Part model, mm, in its own coordinate system. Face numbers are marked on the shaded views. Round coordinates to 2 decimals unless told otherwise and drop trailing zeros. Write each loop counter-clockwise with the first axis right and the second up, starting at its lowest first coordinate (ties: lowest second). Pieces come first, ordered by that corner, then holes.
```python
from build123d import *

# Parameters (mm, degrees)
F0_R     = 13.45
F1_DEPTH = 3


with BuildPart() as f1:
    # F0 (on Front) → F1 (new body)
    with BuildSketch(Plane.XZ):
        with BuildLine():
            ThreePointArc((32.960464, -10.709504), (47.693573, 15.496581), (20.370687, 28.037846))
            ThreePointArc((20.370687, 28.037846), (0, 50.14799), (-20.370687, 28.037846))
            ThreePointArc((-20.370687, 28.037846), (-47.693573, 15.496581), (-32.960464, -10.709504))
            ThreePointArc((-32.960464, -10.709504), (-29.476249, -40.570576), (0, -34.656683))
            ThreePointArc((0, -34.656683), (29.476249, -40.570576), (32.960464, -10.709504))
        make_face()
        with Locations((-17.462441, -24.034988)):
            Circle(F0_R, mode=Mode.SUBTRACT)
        with BuildLine():
            ThreePointArc((-4.876476, 9.860019), (5.803394, 9.34455), (11, 0))
            ThreePointArc((11, 0), (4.993895, -9.801072), (-6.465638, -8.899187))
            ThreePointArc((-6.465638, -8.899187), (-8.321652, -7.193754), (-9.740726, -5.110602))
            ThreePointArc((-9.740726, -5.110602), (-10.960741, -0.928525), (-10.461622, 3.399187))
            ThreePointArc((-10.461622, 3.399187), (-8.321652, 7.193754), (-4.876476, 9.860019))
        make_face(mode=Mode.SUBTRACT)
        with Locations((17.462441, -24.034988)):
            Circle(F0_R, mode=Mode.SUBTRACT)
        with Locations((-28.254823, 9.180549)):
            Circle(F0_R, mode=Mode.SUBTRACT)
        with Locations((0, 29.708879)):
            Circle(F0_R, mode=Mode.SUBTRACT)
        with Locations((28.254823, 9.180549)):
            Circle(F0_R, mode=Mode.SUBTRACT)
    extrude(amount=F1_DEPTH)


solid = f1.part
```
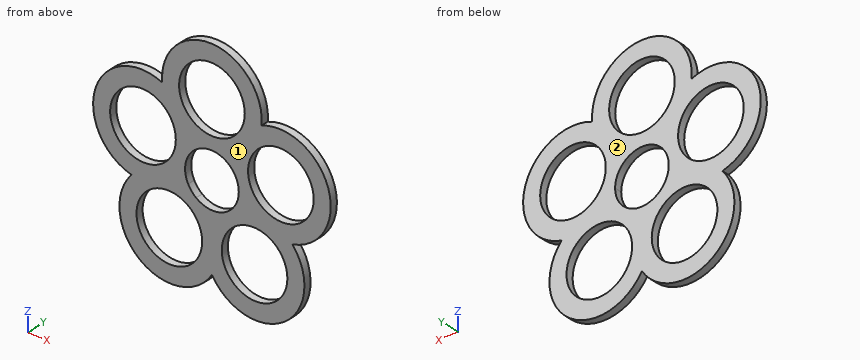
Q1. Cut at C-C on y = -2.2. Write the cut outline in (x, z), plus the area to 3 significant figures.
Values follow:
outline: (-32.96, -10.71) arc R20.44 ccw (long way) to (0, -34.66) arc R20.44 ccw (long way) to (32.96, -10.71) arc R20.44 ccw (long way) to (20.37, 28.04) arc R20.44 ccw (long way) to (-20.37, 28.04) arc R20.44 ccw (long way) to start; hole circle Ø26.9 at (-28.25, 9.18); hole circle Ø26.9 at (-17.46, -24.03); hole circle Ø26.9 at (0, 29.71); hole (-10.46, 3.4) arc R11 ccw to (-9.74, -5.11) arc R11 ccw to (-6.47, -8.9) arc R11 ccw (long way) to (-4.88, 9.86) arc R11 ccw to start; hole circle Ø26.9 at (17.46, -24.03); hole circle Ø26.9 at (28.25, 9.18)
area: 3,260 mm2
Q2. Mould opens along Y. For the marked faces 1 and 2 say: +Y half, -Y half, draft (parallel to the pull), parting line (faces both ways), or undercut.
Values follow:
face 1: -Y half
face 2: +Y half
Q3. Drop flat-ended pins along their axis: pin 1 (1 mm diameter, centred on y = -2.5, z = -27, fed in from +X); pin 2 (1 mm diameter, centred on y = -0.5, z = 28, fed in from -X). Give the stop position or say it passes through.
Values follow:
pin 1: stops at x = 37.75
pin 2: stops at x = -37.32
Q4. Wall check: L1, parallel to X at y = -0.5, z = -24.5; L2, parallel to Z at x = 7, y = -2.35; L3, parallel to Z at x = -3, y = -2. Give the ranges that are in metal, low to high.
Values follow:
L1: x = -37.9 to -30.9, -4.02 to 4.02, 30.9 to 37.9
L2: z = -41.59 to -32.49, -15.58 to -8.49, 8.49 to 18.22, 41.19 to 48.91
L3: z = -38.48 to -10.58, 10.58 to 16.6, 42.82 to 49.93
Q5. Cut at A-A on x = 23. Write the cut outline in (y, z).
Values follow:
outline: (-3, -43.71) - (0, -43.71) - (0, -36.29) - (-3, -36.29) - close; (-3, -11.78) - (0, -11.78) - (0, -3.2) - (-3, -3.2) - close; (-3, 21.56) - (0, 21.56) - (0, 28.93) - (-3, 28.93) - close
Q6. Cut at B-B on x = 9.5. Write the cut outline in (y, z).
Values follow:
outline: (-3, -42.86) - (0, -42.86) - (0, -34.87) - (-3, -34.87) - close; (-3, -13.2) - (0, -13.2) - (0, -5.55) - (-3, -5.55) - close; (-3, 5.55) - (0, 5.55) - (0, 20.19) - (-3, 20.19) - close; (-3, 39.23) - (0, 39.23) - (0, 47.81) - (-3, 47.81) - close
